Autodesk Inventor part; units mm, degrees
ref_plane "YZ Plane" through (0, 0, 0) normal (1, 0, 0) x (0, 1, 0)
ref_plane "XZ Plane" through (0, 0, 0) normal (0, 1, 0) x (-1, 0, 0)
ref_plane "XY Plane" through (0, 0, 0) normal (0, 0, 1) x (1, 0, 0)
sketch "Sketch1" plane through (0, 0, 0) normal (0, 1, 0) x (-1, 0, 0)
  circle A0 centre (0, 0) radius 35
  circle A1 centre (25, 0) radius 4
  dimension "d0" = 70
  dimension "d1" = 8
  dimension "d2" = 25
extrude "Extrusion1" add sketch "Sketch1" along normal blind 2
extrude "Extrusion2" add sketch "Sketch1" along normal blind 25 contours A1
sketch "Sketch2" plane through (0, 2, 0) normal (0, 1, 0) x (1, 0, 0)
  point P0 (0, 0)
sketch "Sketch3" plane through (0, 2, 0) normal (0, 1, 0) x (1, 0, 0)
  circle A0 centre (34, 0) radius 1
  point P0 (0, 0)
  dimension "d7" = 2
  dimension "d8" = 34
extrude "Extrusion3" cut sketch "Sketch3" against normal through all
properties part number "Feul_ClosePlate"
Here's how the part is built. I have some questions about the finished solid (model axes, mm). Round coordinates to 2 decimals unless told otherwise and drop trailing zeros. Order: outer loops, then holes, each group sorted by start corner. A loop starts at its lowest first (then second) coordinate and runs counter-clockwise, first axis right, second up. Notation, with made-up numbers: (59, 60) -> (88, 60) arc R13 ccw to (88, 84) -> close; hole circle Ø11 at (76.5, -23). An arc over 180 degrees is marked (long way). Use CSV: the item, a comma, the result in double quotes.
1. I want a section at C-C on y = 3.75. List the corners of the cut face in (x, z) for me.
Recorded:
outline,"circle Ø8 at (-25, 0)"
2. Thinking about a two-plate mould opening in X: for faces 1 (the face through (0, 2, 0)), 2 (the face through (33.263, 1.014, -0.676)), 3 (the face through (-21.8, 13.3, 2.4)), which applies, pulls with the +X half, pulls with the -X half, needs draft (parallel to the pull), parting line crosses it, or undercut?
Recorded:
face 1,"needs draft"
face 2,"undercut"
face 3,"parting line crosses it"
3. I need wall thicknesses on line 1 along Y through (x, z) = (-23.5, -24.5); line 2 along X through (y, z) = (11.75, -1.5); line 3 along Z through (x, y) = (7.5, 1.75). Which ranges of each line are inside material? Lowest first, please.
Recorded:
line 1,"y = 0 to 2"
line 2,"x = -28.71 to -21.29"
line 3,"z = -34.19 to 34.19"
4. I'm going to push a flat-ended pin straight in: P1, Ø6, axis at y = 8, z = -5, coming from the -X side. Where does the tip first touch, or does it pass through?
Recorded:
P1,"stops at x = -28.46"
5. I want a section at B-B on x = -25. List the corners of the cut face in (y, z) for me, and give its area (3 significant figures).
Recorded:
outline,"(0, -24.49) -> (2, -24.49) -> (2, -4) -> (25, -4) -> (25, 4) -> (2, 4) -> (2, 24.49) -> (0, 24.49) -> close"
area,"282 mm2"
6. I want a section at D-D on z = 26. List the corners of the cut face in (x, y) for me.
Recorded:
outline,"(-23.43, 0) -> (23.43, 0) -> (23.43, 2) -> (-23.43, 2) -> close"
7. I want a section at A-A on x = 34. List the corners of the cut face in (y, z) for me, and give its area (3 significant figures).
Recorded:
outline,"(0, -8.31) -> (2, -8.31) -> (2, -1) -> (0, -1) -> close; (0, 1) -> (2, 1) -> (2, 8.31) -> (0, 8.31) -> close"
area,"29.2 mm2"
